Here's how the part is built. I have some questions about the finished solid (model axes, mm). Round coordinates to 2 decimals unless told otherwise and drop trailing zeros. Order: outer loops, then holes, each group sorted by start corner. A loop starts at its lowest first (then second) coordinate and runs counter-clockwise, first axis right, second up. Notation, with made-up numbers: (-26.5, 44.5) -> (3.5, 44.5) arc R25 ccw to (3.5, 70.5) -> close; hole circle Ø7 at (-19.5, -9). An arc over 180 degrees is marked (long way). Answer in a Markdown table with one row per item.
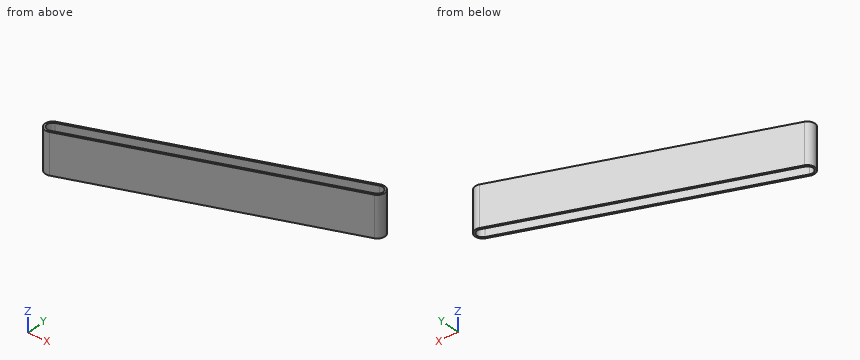
```python
from build123d import *

# Parameters (mm, degrees)
BOSS_EXTRUDE1_DEPTH = 139.7
CUT_EXTRUDE1_DEPTH  = 1903.021697166


with BuildPart() as part:
    # Sketch2 → Boss-Extrude1 (new, symmetric)
    with BuildSketch(Plane.XY):
        with BuildLine():
            Line((-18.425433745, 47.340715999), (1673.352830516, 705.796078626))
            ThreePointArc((1673.352830516, 705.796078626), (1739.11898026, 676.880796373), (1710.203698007, 611.114646628))
            Line((1710.203698007, 611.114646628), (18.425433745, -47.340715999))
            ThreePointArc((18.425433745, -47.340715999), (-47.340715999, -18.425433745), (-18.425433745, 47.340715999))
        make_face()
    extrude(amount=BOSS_EXTRUDE1_DEPTH, both=True)

    # Sketch7 → Cut-Extrude1 (cut, through all)
    with BuildSketch(Plane.XY.offset(139.7)):
        with BuildLine():
            Line((13.819075309, -35.505536999), (1705.59733957, 622.949825628))
            ThreePointArc((1705.59733957, 622.949825628), (1727.283801261, 672.274437937), (1677.959188952, 693.960899627))
            Line((1677.959188952, 693.960899627), (-13.819075309, 35.505536999))
            ThreePointArc((-13.819075309, 35.505536999), (-35.505536999, -13.819075309), (13.819075309, -35.505536999))
        make_face()
    extrude(amount=-CUT_EXTRUDE1_DEPTH, mode=Mode.SUBTRACT)


solid = part.part
```
1. Suppose I cut it at B-B on x = 1121. Write out the boundary of the cut face in (y, z), then the cut area to 3 significant figures.
Numbers:
| item | result |
|---|---|
| outline | (381.79, -139.7) -> (395.42, -139.7) -> (395.42, 139.7) -> (381.79, 139.7) -> close; (477.19, -139.7) -> (490.82, -139.7) -> (490.82, 139.7) -> (477.19, 139.7) -> close |
| area | 7,620 mm2 |
2. Suppose I cut it at A-A on z = 113. Write out the boundary of the cut face in (x, y).
Numbers:
| item | result |
|---|---|
| outline | (-18.43, 47.34) arc R50.8 ccw to (18.43, -47.34) -> (1710.2, 611.11) arc R50.8 ccw to (1673.35, 705.8) -> close; hole (-13.82, 35.51) arc R38.1 ccw to (13.82, -35.51) -> (1705.6, 622.95) arc R38.1 ccw to (1677.96, 693.96) -> close |
3. For pin 1 Ø4 at (x, z) = (847, 25.5) entering from -Y; pin 2 Ø1.5 at (x, z) = (728.5, 98) entering from -Y; pin 3 Ø1 at (x, z) = (417.5, 101.5) entering from +Y, each with a flat end and sliding along its axis, tell me the tip position at first contact or that it passes through.
Numbers:
| item | result |
|---|---|
| pin 1 | stops at y = 274.37 |
| pin 2 | stops at y = 228.73 |
| pin 3 | stops at y = 217.2 |
4. Suppose I cut it at C-C on y = 0. Write out the boundary of the cut face in (x, z).
Numbers:
| item | result |
|---|---|
| outline | (-50.8, -139.7) -> (-38.1, -139.7) -> (-38.1, 139.7) -> (-50.8, 139.7) -> close; (105.04, -139.7) -> (140.06, -139.7) -> (140.06, 139.7) -> (105.04, 139.7) -> close |
5. Please list where these lines run through material, in increasing order: line 1 along Y through (x, z) = (652, 104); line 2 along Y through (x, z) = (1641.5, -34).
Numbers:
| item | result |
|---|---|
| line 1 | y = 199.25 to 212.88, 294.65 to 308.28 |
| line 2 | y = 584.37 to 598, 679.77 to 693.4 |
